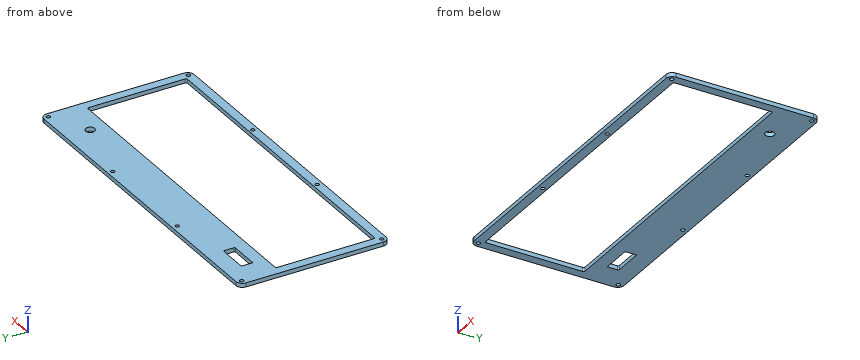
```python
from build123d import *

# Parameters (mm, degrees)
SKETCH_W        = 263.525
SKETCH_H        = 117.475
PAD_DEPTH       = 3.175
SKETCH002_W     = 249.2375
SKETCH002_H     = 77.7875
POCKET_DEPTH    = 3.176
SKETCH003_R     = 3.6
POCKET001_DEPTH = 3.176
SKETCH001_R     = 1.5494
HOLE_DEPTH      = 3.176
FILLET_R        = 5.08
FILLET001_R     = 1.27
SKETCH004_W     = 23.715193
SKETCH004_H     = 9.0125
POCKET002_DEPTH = 3.176
FILLET002_R     = 0.79375


with BuildPart() as part:
    # Sketch → Pad (new body)
    with BuildSketch(Plane.XY):
        Rectangle(SKETCH_W, SKETCH_H)
    extrude(amount=PAD_DEPTH)

    # Sketch002 (on Face6 of Pad) → Pocket (cut, through all)
    with BuildSketch(Plane.XY.offset(3.175)):
        with Locations((0, -12.7)):
            Rectangle(SKETCH002_W, SKETCH002_H)
    extrude(amount=-POCKET_DEPTH, mode=Mode.SUBTRACT)

    # Sketch003 (on Face5 of Pocket) → Pocket001 (cut, through all)
    with BuildSketch(Plane.XY.offset(3.175)):
        with Locations((98.425, 39.37)):
            Circle(SKETCH003_R)
    extrude(amount=-POCKET001_DEPTH, mode=Mode.SUBTRACT)

    # Sketch001 (on Face6 of Pad) → Hole (cut, through all)
    with BuildSketch(Plane.XY.offset(3.175)):
        with Locations((-42.597917, 54.76875)):
            Circle(SKETCH001_R)
        with Locations((42.597917, 54.76875)):
            Circle(SKETCH001_R)
        with Locations((42.597917, -54.76875)):
            Circle(SKETCH001_R)
        with Locations((-42.597917, -54.76875)):
            Circle(SKETCH001_R)
        with Locations((-127.79375, -54.76875)):
            Circle(SKETCH001_R)
        with Locations((-127.79375, 54.76875)):
            Circle(SKETCH001_R)
        with Locations((127.79375, 54.76875)):
            Circle(SKETCH001_R)
        with Locations((127.79375, -54.76875)):
            Circle(SKETCH001_R)
    extrude(amount=-HOLE_DEPTH, mode=Mode.SUBTRACT)

    # Fillet
    fillet_edges = [part.edges().sort_by_distance(p)[0] for p in [
        (-131.7625, 58.7375, 1.5875),
        (-131.7625, -58.7375, 1.5875),
        (131.7625, -58.7375, 1.5875),
        (131.7625, 58.7375, 1.5875),
    ]]
    fillet(fillet_edges, radius=FILLET_R)

    # Fillet001
    fillet001_edges = [part.edges().sort_by_distance(p)[0] for p in [
        (-124.61875, -51.59375, 1.5875),
        (-124.61875, 26.19375, 1.5875),
        (124.61875, 26.19375, 1.5875),
        (124.61875, -51.59375, 1.5875),
    ]]
    fillet(fillet001_edges, radius=FILLET001_R)

    # Sketch004 (on Face5 of Pocket001) → Pocket002 (cut, through all)
    with BuildSketch(Plane.XY.offset(3.175)):
        with Locations((-98.975303, 40.54573)):
            Rectangle(SKETCH004_W, SKETCH004_H)
    extrude(amount=-POCKET002_DEPTH, mode=Mode.SUBTRACT)

    # Fillet002
    fillet002_edges = [part.edges().sort_by_distance(p)[0] for p in [
        (-110.8329, 45.05198, 1.5875),
        (-87.117707, 45.05198, 1.5875),
        (-87.117707, 36.03948, 1.5875),
        (-110.8329, 36.03948, 1.5875),
    ]]
    fillet(fillet002_edges, radius=FILLET002_R)


solid = part.part
```
Can you work these out from the model? Positions are in its coordinate system, mm. Give positions to 0.01 mm unless a question says otherwise; leave off trailing zeros. Write each loop counter-clockwise with the first axis right and the second up, starting at its lowest first coordinate (ties: lowest second). Pieces come first, ordered by that corner, then holes. Notation, with made-up numbers: (-39, -38.5) - (-13, -38.5) arc R12 ccw to (-13, -23.5) - close; hole circle Ø2 at (-7.75, 26.5). An arc over 180 degrees is marked (long way). Write item = value, one per line. Start each with the question number.
1. Imagine slicing it at A-A (x = 75.5). Please give me the cut outline in (y, z) (1 decimal), and give its area (3 significant figures).
2. For pin 1 (1.9 mm diameter, centred on x = 127.79, y = -54.77, fed in from +Z), with a flat end and sliding along its axis, tell me the tip position at first contact or that it passes through.
3. Imagine slicing it at D-D (z = 2.25). Count the separate pieces of the cut face and the enclosed holes in it, and give its area (3 significant figures).
4. Please list where these lines run through material, in increasing order: line 1 (Y direction, x = -78, z = 2.8); line 2 (X direction, y = 24.5, z = 0.45); line 3 (X direction, y = 38, z = 2.5).
5. Imagine slicing it at C-C (y = 39.37). Please give me the cut outline in (x, z) (1 decimal).
6. Imagine slicing it at B-B (y = 10). Please give me the cut outline in (x, z) (1 decimal).
Worked answers:
q1.outline = (-58.7, 0) - (-51.6, 0) - (-51.6, 3.2) - (-58.7, 3.2) - close; (26.2, 0) - (58.7, 0) - (58.7, 3.2) - (26.2, 3.2) - close
q1.area = 126 mm2
q2.pin_1 = through
q3.separate_pieces = 1
q3.enclosed_holes = 11
q3.area = 11,200 mm2
q4.line_1 = -58.74 to -51.59, 26.19 to 58.74
q4.line_2 = -131.76 to -124.62, 124.62 to 131.76
q4.line_3 = -131.76 to -110.83, -87.12 to 95.1, 101.75 to 131.76
q5.outline = (-131.8, 0) - (-110.8, 0) - (-110.8, 3.2) - (-131.8, 3.2) - close; (-87.1, 0) - (94.8, 0) - (94.8, 3.2) - (-87.1, 3.2) - close; (102, 0) - (131.8, 0) - (131.8, 3.2) - (102, 3.2) - close
q6.outline = (-131.8, 0) - (-124.6, 0) - (-124.6, 3.2) - (-131.8, 3.2) - close; (124.6, 0) - (131.8, 0) - (131.8, 3.2) - (124.6, 3.2) - close
